The model under review builds one solid part; all positions refer to its coordinate system, in mm. A direction names the side the tool comes from. Give positions to 0.01 mm unless a question says otherwise; leave off trailing zeros. Loops run counter-clockwise (first coordinate to the right, second up) from the corner with the lowest first, then second, coordinate; pieces in that order, holes last. Notation, with made-up numbers: (-20.75, -24.75) - (18.25, -24.75) arc R35 ccw to (18.25, 9.25) - close; hole circle Ø9 at (-27, 9). An arc over 180 degrees is marked (long way). Return JSON: item names as keys, results as strings. Group by question number.
from build123d import *

# Parameters (mm, degrees)
F0_R     = 2.75
F1_DEPTH = 1.5
F2_R     = 16.75
F3_DEPTH = 2
F2_R_2   = 2.75
F5_DEPTH = 2.5
F6_R     = 16.75
F6_R_2   = 16.25
F7_DEPTH = 3
F8_SIZE  = 1
F9_R     = 0.5


# Not quite as in the source:
# - a feature names something its author has since deleted; it is built from what else it names


with BuildPart() as f1:
    # F0 (on Top) → F1 (new body)
    with BuildSketch(Plane.XY):
        with BuildLine():
            ThreePointArc((-8.6418314576, 15.5042332625), (-8.9908284276, -15.3044929412), (17.75, 0))
            ThreePointArc((17.75, 0), (15.3044929412, 8.9908284276), (8.6418314576, 15.5042332625))
            ThreePointArc((8.6418314576, 15.5042332625), (0, 17.75), (-8.6418314576, 15.5042332625))
        make_face()
        with BuildLine():
            ThreePointArc((-8.6418314576, 15.5042332625), (0, 17.75), (8.6418314576, 15.5042332625))
            ThreePointArc((8.6418314576, 15.5042332625), (6.5916833801, 22.4532341762), (0, 25.4601314234))
            ThreePointArc((0, 25.4601314234), (-6.5916833801, 22.4532341762), (-8.6418314576, 15.5042332625))
        make_face()
        with Locations((0, 21.05)):
            Circle(F0_R, mode=Mode.SUBTRACT)
    extrude(amount=F1_DEPTH)

    # F2 (on face) → F3 (join)
    with BuildSketch(Plane.XY.offset(1.5)):
        with BuildLine():
            ThreePointArc((-8.6418314576, 15.5042332625), (-8.9908284276, -15.3044929412), (17.75, 0))
            ThreePointArc((17.75, 0), (15.3044929412, 8.9908284276), (8.6418314576, 15.5042332625))
            ThreePointArc((8.6418314576, 15.5042332625), (0, 17.75), (-8.6418314576, 15.5042332625))
        make_face()
        Circle(F2_R, mode=Mode.SUBTRACT)
    extrude(amount=F3_DEPTH)

    # F2 (on face) → F5 (join)
    with BuildSketch(Plane.XY.offset(1.5)):
        with BuildLine():
            ThreePointArc((-8.6418314576, 15.5042332625), (0, 17.75), (8.6418314576, 15.5042332625))
            ThreePointArc((8.6418314576, 15.5042332625), (0, 25.4601314234), (-8.6418314576, 15.5042332625))
        make_face()
        with Locations((0, 21.05)):
            Circle(F2_R_2, mode=Mode.SUBTRACT)
    extrude(amount=F5_DEPTH)

    # F6 (on face) → F7 (join)
    with BuildSketch(Plane.XY.offset(3.5)):
        with BuildLine():
            ThreePointArc((-8.6418314576, 15.5042332625), (-8.9908284276, -15.3044929412), (17.75, 0))
            ThreePointArc((17.75, 0), (15.3044929412, 8.9908284276), (8.6418314576, 15.5042332625))
            ThreePointArc((8.6418314576, 15.5042332625), (0, 17.75), (-8.6418314576, 15.5042332625))
        make_face()
        Circle(F6_R, mode=Mode.SUBTRACT)
        Circle(F6_R)
        Circle(F6_R_2, mode=Mode.SUBTRACT)
    extrude(amount=F7_DEPTH)

    # F8
    f8_edges = [f1.edges().sort_by_distance(p)[0] for p in [
        (-16.25, 0, 6.5),
    ]]
    chamfer(f8_edges, length=F8_SIZE)

    # F9
    f9_edges = [f1.edges().sort_by_distance(p)[0] for p in [
        (-2.75, 21.05, 0),
    ]]
    fillet(f9_edges, radius=F9_R)


solid = f1.part
Item 1: Take a section at B-B (z = 4.5). State the section outline as (x, y) points.
Item 2: Tool access review of faces 1 (the face through (-2.6, 16.2, 3.5)), 2 (the face through (15.5, 4.88, 4.49)), 3 (the face through (0, -1, 0)): name each direction out of +Z, -Z, +X, -X, +Y, -Y from which nothing blocks a thin tool from reaching the whole face with its end or side.
Item 3: Take a section at A-A (y = 0). State the section outline as (x, z) points, then the cut area to 4 significant figures.
Item 4: Mouldability with a two-part tool opening along X and no side actions: class faces 4 (the face through (-3.63, -16.35, 2.49)), 5 (the face through (0, 0, 1.5)), 6 (the face through (-15, 9, 6.5)), 7 (the face through (8.191, -15.747, 3.204)) as +X half, -X half, draft (parallel to the pull), parting line (faces both ways), or undercut.
Item 5: For L1, parallel to Y at x = 0, z = 2.6; L2, parallel to Y at x = 0, z = 4.65; L3, parallel to Y at x = 1.5, z = 2, list the stretches that pass through material, from the lowest coordinate up. Write a range as from..to.
Item 6: For P1, Ø8, axis at x = -3, y = 22, coming from the +Z side; P2, Ø1, axis at x = 13.5, z = 5.5, coming from the -Y side; P3, Ø1, axis at y = 4.5, z = 3, coming from the +X side, all flat-tipped, find the tip position at first contact; note any pin that passes through.
Check sheet entries:
{
 "1": {"outline": "circle Ø35.5 at (0, 0); hole circle Ø32.5 at (0, 0)"},
 "2": {"face 1": "none", "face 2": "+Z", "face 3": "-Z, +X, -X, +Y, -Y"},
 "3": {"outline": "(-17.75, 0) - (17.75, 0) - (17.75, 6.5) - (17.25, 6.5) - (16.25, 5.5) - (16.25, 3.5) - (16.75, 3.5) - (16.75, 1.5) - (-16.75, 1.5) - (-16.75, 3.5) - (-16.25, 3.5) - (-16.25, 5.5) - (-17.25, 6.5) - (-17.75, 6.5) - close", "area": "65.25 mm^2"},
 "4": {"face 4": "undercut", "face 5": "undercut", "face 6": "draft", "face 7": "parting line"},
 "5": {"L1": "y = -17.75..-16.75, 16.75..18.3, 23.8..25.46", "L2": "y = -17.75..-16.25, 16.25..17.75", "L3": "y = -17.69..-16.68, 16.68..18.75, 23.35..25.33"},
 "6": {"P1": "stops at z = 4", "P2": "stops at y = -12.09", "P3": "stops at x = 17.29"}
}
